Check sheet for the modelled part. Datum: model origin and axes. Units: mm. Face numbers are marked on the shaded views. A direction names the side the tool comes from. Round coordinates to 2 decimals unless told otherwise and drop trailing zeros. Loops run counter-clockwise (first coordinate to the right, second up) from the corner with the lowest first, then second, coordinate; pieces in that order, holes last. Notation, with made-up numbers: (14.25, 71) -> (55.25, 71) arc R29 cw to (55.25, 99) -> close; hole circle Ø1 at (-14, 48.5). An arc over 180 degrees is marked (long way). Return JSON: item names as keys, results as strings.
Autodesk Inventor part; units mm, degrees
ref_plane "YZ Plane" through (0, 0, 0) normal (1, 0, 0) x (0, 1, 0)
ref_plane "XZ Plane" through (0, 0, 0) normal (0, 1, 0) x (-1, 0, 0)
ref_plane "XY Plane" through (0, 0, 0) normal (0, 0, 1) x (1, 0, 0)
sketch "Sketch1" plane through (0, 0, 0) normal (0, 0, 1) x (1, 0, 0)
  line L0 (-30, 32.5) -> (30, 32.5)
  line L1 (30, 32.5) -> (30, -32.5)
  line L2 (30, -32.5) -> (-30, -32.5)
  line L3 (-30, -32.5) -> (-30, 32.5)
  point P0 (0, 0)
  point P1 (0, 32.5)
  point P2 (-30, 0)
  dimension "d0" = 60
  dimension "d1" = 65
extrude "Extrusion1" add sketch "Sketch1" along normal blind 8
sketch "Sketch4" plane through (0, 0, 8) normal (0, 0, 1) x (1, 0, 0)
  circle A0 centre (-25, -15) radius 1.75
  circle A1 centre (25, -15) radius 1.75
  circle A2 centre (25, -25) radius 1.75
  arc A3 (-10.5, -30) -> (10.5, -30) centre (0, -30) ccw
  line L0 (10.5, -30) -> (10.5, -25)
  arc A4 (10.5, -25) -> (-10.5, -25) centre (0, -25) ccw
  line L1 (-10.5, -25) -> (-10.5, -30)
  line L2 (30, -10) -> (30, -50)
  line L3 (30, -50) -> (-30, -50)
  line L4 (-30, -50) -> (-30, -10)
  line L5 (-30, -10) -> (30, -10)
  line L6 (25, -27.5) -> (25, -22.5) construction
  line L7 (26.75, -27.5) -> (26.75, -22.5)
  line L8 (23.25, -22.5) -> (23.25, -27.5)
  arc A5 (23.25, -27.5) -> (26.75, -27.5) centre (25, -27.5) ccw
  arc A6 (26.75, -22.5) -> (23.25, -22.5) centre (25, -22.5) ccw
  line L9 (-25, -27.5) -> (-25, -22.5) construction
  line L10 (-23.25, -27.5) -> (-23.25, -22.5)
  line L11 (-26.75, -22.5) -> (-26.75, -27.5)
  arc A7 (-26.75, -27.5) -> (-23.25, -27.5) centre (-25, -27.5) ccw
  arc A8 (-23.25, -22.5) -> (-26.75, -22.5) centre (-25, -22.5) ccw
  line L12 (-30, -32.5) -> (30, -32.5)
  point P0 (0, 0)
  point P1 (-25, -25)
  point P2 (26.75, -25)
  point P3 (23.25, -25)
  dimension "d22" = 5
  dimension "d23" = 3.5
  dimension "d24" = 5
  dimension "d25" = 10.5
  dimension "d26" = 7.5
  dimension "d27" = 30
extrude "Extrusion4" cut sketch "Sketch4" against normal blind 10 contours A2 | L7 A5 L8 A2 | A2 L8 A6 L7 | L1 A4 L0 A3 L12 | L12 A3 | A7 L11 A8 L10
sketch "Sketch5" plane through (0, 0, 8) normal (0, 0, 1) x (1, 0, 0)
  circle A0 centre (10, 6.8914) radius 7.5
  line L0 (30, 32.5) -> (-30, 32.5)
  line L1 (30, -32.5) -> (30, 32.5)
  point P0 (0, 0)
  dimension "d13" = 15
  dimension "d28" = 25.6086
  dimension "d29" = 20
extrude "Extrusion5" cut sketch "Sketch5" against normal through all
sketch "Sketch6" plane through (0, 0, 8) normal (0, 0, 1) x (1, 0, 0)
  circle A0 centre (20, 17.6414) radius 1.75
  circle A1 centre (0, 17.6414) radius 1.75
  circle A2 centre (0, -3.8586) radius 1.75
  circle A3 centre (20, -3.8586) radius 1.75
  line L0 (0, 17.6414) -> (20, 17.6414) construction
  line L1 (20, 17.6414) -> (20, -3.8586) construction
  line L2 (20, -3.8586) -> (0, -3.8586) construction
  line L3 (0, -3.8586) -> (0, 17.6414) construction
  line L4 (30, -32.5) -> (30, 32.5) construction
  line L5 (30, 32.5) -> (-30, 32.5) construction
  circle A4 centre (10, 6.8914) radius 7.5
  point P0 (0, 0)
  point P1 (10, -3.8586)
  point P2 (20, 6.8914)
  dimension "d31" = 21.5
  dimension "d33" = 3.5
  dimension "d42" = 20
extrude "Extrusion6" cut sketch "Sketch6" against normal through all contours A0 | A1 | A2 | A3
sketch "Sketch7" plane through (0, 0, 8) normal (0, 0, 1) x (1, 0, 0)
  line L0 (-30, 32.5) -> (-30, -32.5)
  line L1 (-30, -7.5) -> (-25, -7.5)
  line L2 (-25, -7.5) -> (-25, 32.5)
  line L3 (-25, 32.5) -> (-30, 32.5)
  line L4 (-30, 32.5) -> (-30, -7.5)
  line L5 (30, 32.5) -> (-30, 32.5)
  line L6 (30, -10) -> (-30, -10)
  line L7 (25, -10) -> (30, -10)
  line L8 (30, -10) -> (30, 32.5)
  line L9 (30, 32.5) -> (25, 32.5)
  line L10 (25, 32.5) -> (25, -10)
  line L11 (30, -32.5) -> (30, 32.5)
  point P0 (0, 0)
  point P1 (25, -10)
  dimension "d18" = 5
  dimension "d19" = 5
  dimension "d43" = 40
extrude "Extrusion7" cut sketch "Sketch7" against normal through all contours L3 L2 L1 L0 | L5 L8 L6 L10
sketch "Sketch8" plane through (0, 0, 8) normal (0, 0, 1) x (1, 0, 0)
  circle A0 centre (-13, 5.0309) radius 4
  line L0 (-30, -7.5) -> (-30, -32.5)
  line L1 (25, 32.5) -> (-25, 32.5)
  point P0 (0, 0)
  dimension "d35" = 8
  dimension "d36" = 17
  dimension "d37" = 27.4691
extrude "Extrusion8" cut sketch "Sketch8" against normal blind 10
move faces "Move1" translate (0, 8, 0) faces at (8.3333, 32.5, 2.6667)
sketch "Sketch9" plane through (0, 0, 0) normal (0, 0, -1) x (-1, 0, 0)
  line L0 (-25, 40.5) -> (25, 40.5)
  point P0 (0, 0)
  point P1 (0, 36.5)
  point P2 (-20, 36.5)
  point P3 (20, 36.5)
  dimension "d47" = 20
  dimension "d48" = 20
  dimension "d49" = 4
hole "Hole1" at (0, 36.5, 0) at (20, 36.5, 0) at (-20, 36.5, 0) direction (0, 0, 1) diameter 4.5 end through all
fillet "Fillet1" radius 1.5 2 edges at (25, -10, 4) (-25, -7.5, 4)
equation "\"d19\" = d18"
properties part number "0005-10-005"
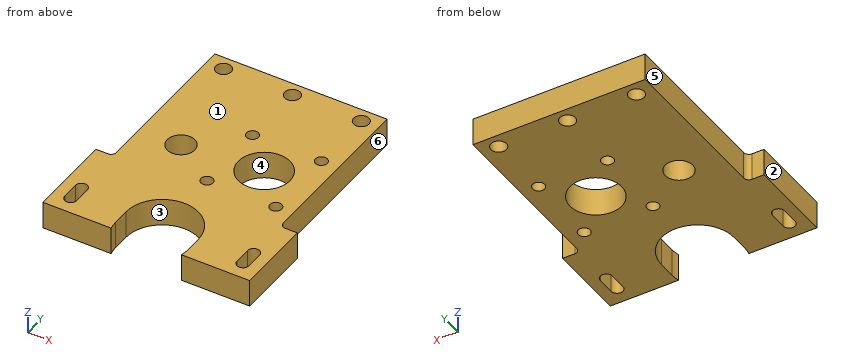
Q1. Tool access check on the marked faces 4, 5 and 6. Record the directions out of +Z, -Z, +X, -X, +Y, -Y that give a thin tool (end or side, any length) a straight path to the whole face; none if there is none.
Results list:
{"face 4": "+Z, -Z", "face 5": "+Z, -Z, -X, +Y", "face 6": "+Z, -Z, +X, +Y"}
Q2. Section check C-C (y = 10.5). Record the boundary of the cut face in (x, z).
Results list:
{"outline": "(-25, 0) -> (3.43, 0) -> (3.43, 8) -> (-25, 8) -> close; (16.57, 0) -> (25, 0) -> (25, 8) -> (16.57, 8) -> close"}
Q3. Section check B-B (y = 36.5). Record the boundary of the cut face in (x, z).
Results list:
{"outline": "(-25, 0) -> (-22.25, 0) -> (-22.25, 8) -> (-25, 8) -> close; (-17.75, 0) -> (-2.25, 0) -> (-2.25, 8) -> (-17.75, 8) -> close; (2.25, 0) -> (17.75, 0) -> (17.75, 8) -> (2.25, 8) -> close; (22.25, 0) -> (25, 0) -> (25, 8) -> (22.25, 8) -> close"}
Q4. Go/stop test with flat-tipped pins: pin 1 (1.8 mm diameter, centred on x = 28.5, z = 5.5, fed in from +Y); pin 2 (4 mm diameter, centred on y = 23, z = 3.5, fed in from -X); pin 3 (4 mm diameter, centred on x = -28.5, z = 5.5, fed in from +Y). Record where each tip stops, or that it passes through.
Results list:
{"pin 1": "y = -10", "pin 2": "x = -25", "pin 3": "y = -7.5"}
Q5. Material ranges on line 1 (Y direction, x = 20, z = 4.75); line 2 (X direction, y = 36.5, z = 6); line 3 (X direction, y = -29, z = 5), recorded low to high.
Results list:
{"line 1": "-32.5 to -5.61, -2.11 to 15.89, 19.39 to 34.25, 38.75 to 40.5", "line 2": "-25 to -22.25, -17.75 to -2.25, 2.25 to 17.75, 22.25 to 25", "line 3": "-30 to -25.9, -24.1 to -10.5, 10.5 to 24.1, 25.9 to 30"}
Q6. Section check D-D (z = 1.75). Count the separate pieces of the cut face and the enclosed holes in it, then the cut area to 3 significant figures.
Results list:
{"separate pieces": "1", "enclosed holes": "11", "area": "3,190 mm^2"}
Q7. Draft check along X on the marked faces 1, 2 and 3. Enter one of: released by +X, released by -X, zero draft, split by the parting line, or undercut.
Results list:
{"face 1": "zero draft", "face 2": "released by -X", "face 3": "undercut"}
Q8. Section check A-A (x = 0). Record the boundary of the cut face in (y, z).
Results list:
{"outline": "(-14.5, 0) -> (-5.61, 0) -> (-5.61, 8) -> (-14.5, 8) -> close; (-2.11, 0) -> (15.89, 0) -> (15.89, 8) -> (-2.11, 8) -> close; (19.39, 0) -> (34.25, 0) -> (34.25, 8) -> (19.39, 8) -> close; (38.75, 0) -> (40.5, 0) -> (40.5, 8) -> (38.75, 8) -> close"}
